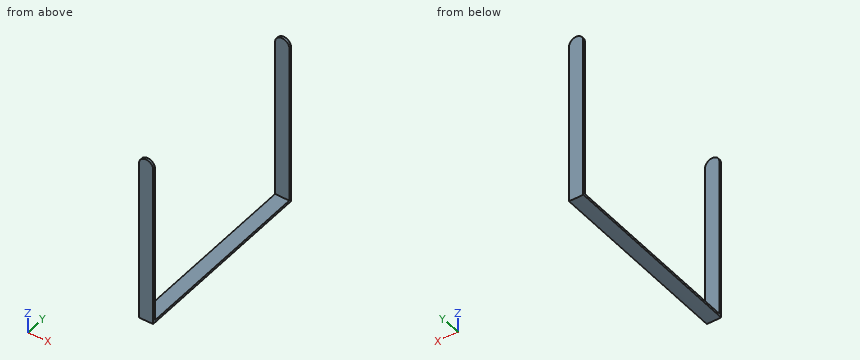
from build123d import *

# Parameters (mm, degrees)
BOSS_EXTRUDE1_DEPTH = 2.54
BOSS_EXTRUDE2_DEPTH = 203.2
BOSS_EXTRUDE3_DEPTH = 2.54


with BuildPart() as part:
    # Sketch1 → Boss-Extrude1 (new body)
    with BuildSketch(Plane(origin=(0, 0, 0), x_dir=(1, 0, 0), z_dir=(0, 1, 0))):
        with BuildLine():
            Line((-7.755527074, 0), (-7.755527074, 177.630773797))
            ThreePointArc((-7.755527074, 177.630773797), (0, 177.8), (7.755527074, 177.630773797))
            Line((7.755527074, 177.630773797), (7.755527074, 0))
            ThreePointArc((7.755527074, 0), (0, -7.755527074), (-7.755527074, 0))
        make_face()
    extrude(amount=BOSS_EXTRUDE1_DEPTH)

    # Sketch2 → Boss-Extrude2 (add)
    with BuildSketch(Plane(origin=(0, 2.54, 0), x_dir=(1, 0, 0), z_dir=(0, 1, 0))):
        with BuildLine():
            Line((-7.755527074, 177.630773797), (-7.755527074, 175.090773797))
            ThreePointArc((-7.755527074, 175.090773797), (0, 175.262452537), (7.755527074, 175.090773797))
            Line((7.755527074, 175.090773797), (7.755527074, 177.630773797))
            ThreePointArc((7.755527074, 177.630773797), (0, 177.8), (-7.755527074, 177.630773797))
        make_face()
    extrude(amount=BOSS_EXTRUDE2_DEPTH)

    # Sketch3 → Boss-Extrude3 (add)
    with BuildSketch(Plane(origin=(0, 205.74, 0), x_dir=(1, 0, 0), z_dir=(0, 1, 0))):
        with BuildLine():
            Line((-7.755527074, 0), (-7.755527074, 177.630773797))
            ThreePointArc((-7.755527074, 177.630773797), (0, 177.8), (7.755527074, 177.630773797))
            Line((7.755527074, 177.630773797), (7.755527074, 0))
            ThreePointArc((7.755527074, 0), (0, -7.755527074), (-7.755527074, 0))
        make_face()
    extrude(amount=BOSS_EXTRUDE3_DEPTH)


solid = part.part
Model file for the job. Use its own axes, mm. Give positions to 0.01 mm unless a question says otherwise; leave off trailing zeros. Order: outer loops, then holes, each group sorted by start corner. A loop starts at its lowest first (then second) coordinate and runs counter-clockwise, first axis right, second up. Notation, with made-up numbers: (24, 53.5) - (48, 53.5) arc R34 ccw to (48, 89.5) - close; hole circle Ø11 at (29, 12.5). An arc over 180 degrees is marked (long way). Return JSON: item names as keys, results as strings.
1) Cut at B-B, the plane x = 0. Give the cut face in (y, z), plus the area to 3 significant figures.
Geometry says:
{"outline": "(0, -177.8) - (208.28, -177.8) - (208.28, 7.76) - (205.74, 7.76) - (205.74, -175.26) - (2.54, -175.26) - (2.54, 7.76) - (0, 7.76) - close", "area": "1,460 mm²"}
2) Probe line 1 (Y direction, x = 2, z = -5); line 2 (Z direction, x = 2.5, y = 149.5); line 3 (Z direction, x = -7, y = 130.5). List the from-to ranges inside material, lowest first. Write a range as from..to.
Geometry says:
{"line 1": "0..2.54, 205.74..208.28", "line 2": "-177.78..-175.24", "line 3": "-177.66..-175.12"}
3) Cut at C-C, the plane y = 19.5. Give the cut face in (x, z).
Geometry says:
{"outline": "(-7.76, -177.63) arc R177.8 ccw to (7.76, -177.63) - (7.76, -175.09) arc R175.26 cw to (-7.76, -175.09) - close"}
4) Cut at A-A, the plane z = -51. Give the cut face in (x, y), plus the area to 3 significant figures.
Geometry says:
{"outline": "(-7.76, 0) - (7.76, 0) - (7.76, 2.54) - (-7.76, 2.54) - close; (-7.76, 205.74) - (7.76, 205.74) - (7.76, 208.28) - (-7.76, 208.28) - close", "area": "78.8 mm²"}
